Answer from the drawing. Dimensions are ordinates in mm from the lowest x, y and z of the part. Coordinates: 2 decimals unless noted, no trailing zeros. Order: outer loops, then holes, each group sorted by start corner. A loop starts at its lowest first (then second) coordinate and runs counter-clockwise, first axis right, second up.
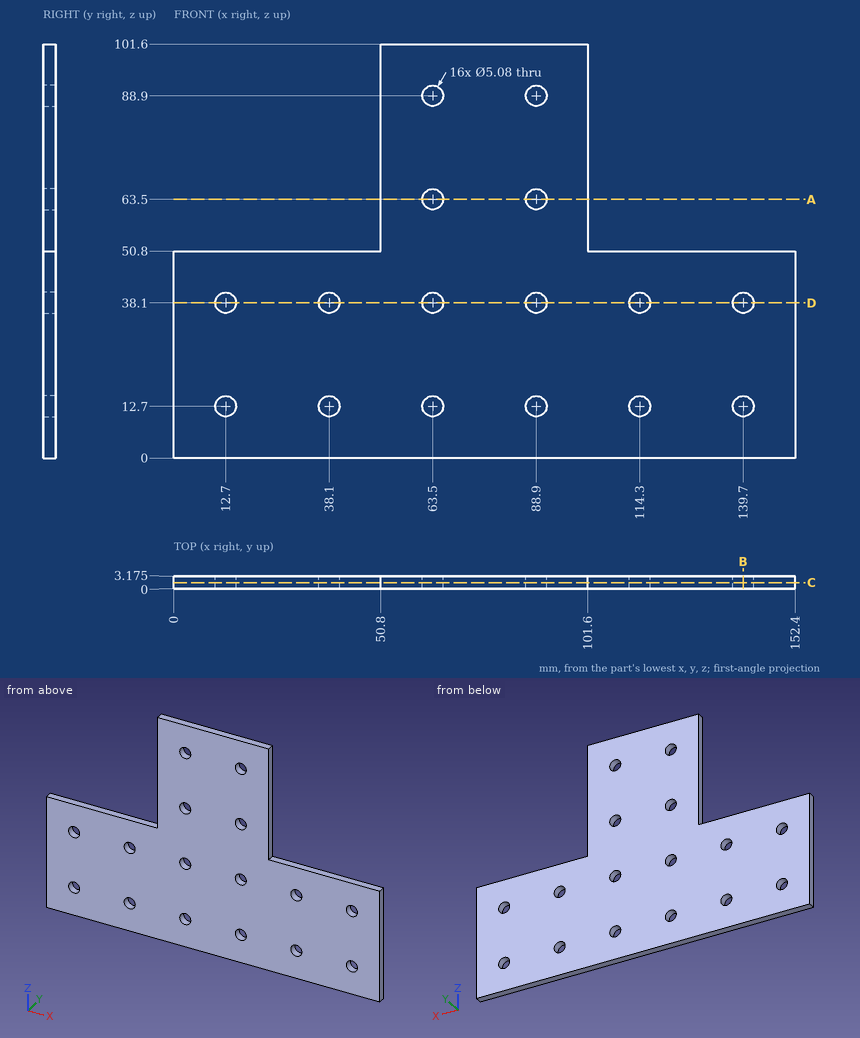
1. Flat-ended cylindrical pins translate along their axes: pin 1 (1 mm diameter, centred on x = 123.5, y = 1, fed in from +Z); pin 2 (3 mm diameter, centred on x = 139.7, z = 38.1, fed in from -Y); pin 3 (1.6 mm diameter, centred on y = 2, z = 68.5, fed in from +X). Find the tip coordinate at first contact, or state that the pin passes through.
2. Consider probe 1 along Z at (x, y) = (13, 1.25); probe 2 along Z at (x, y) = (89.5, 2.1); probe 3 along Z at (x, y) = (45, 1.9). Determine where each line is inside the solid, lowest interval first.
3. The part is cut by section B-B (x = 139.7). Determine the outline of the cut face in (y, z) (3 decimals), plus the area to 3 significant figures.
4. The part is cut by section D-D (z = 38.1). Determine the outline of the cut face in (x, y) (3 decimals).
5. The part is cut by section C-C (y = 1.55). Count the separate pieces of the cut face and the enclosed holes in it, plus the area to 4 significant figures.
6. The part is cut by section A-A (z = 63.5). Determine the outline of the cut face in (x, y) (3 decimals).
Worked out:
1. pin 1: stops at z = 50.8
1. pin 2: passes through
1. pin 3: stops at x = 101.6
2. probe 1: z = 0 to 10.18, 15.22 to 35.58, 40.62 to 50.8
2. probe 2: z = 0 to 10.23, 15.17 to 35.63, 40.57 to 61.03, 65.97 to 86.43, 91.37 to 101.6
2. probe 3: z = 0 to 50.8
3. outline: (0, 0) - (3.175, 0) - (3.175, 10.16) - (0, 10.16) - close; (0, 15.24) - (3.175, 15.24) - (3.175, 35.56) - (0, 35.56) - close; (0, 40.64) - (3.175, 40.64) - (3.175, 50.8) - (0, 50.8) - close
3. area: 129 mm2
4. outline: (0, 0) - (10.16, 0) - (10.16, 3.175) - (0, 3.175) - close; (15.24, 0) - (35.56, 0) - (35.56, 3.175) - (15.24, 3.175) - close; (40.64, 0) - (60.96, 0) - (60.96, 3.175) - (40.64, 3.175) - close; (66.04, 0) - (86.36, 0) - (86.36, 3.175) - (66.04, 3.175) - close; (91.44, 0) - (111.76, 0) - (111.76, 3.175) - (91.44, 3.175) - close; (116.84, 0) - (137.16, 0) - (137.16, 3.175) - (116.84, 3.175) - close; (142.24, 0) - (152.4, 0) - (152.4, 3.175) - (142.24, 3.175) - close
5. separate pieces: 1
5. enclosed holes: 16
5. area: 10,000 mm2
6. outline: (50.8, 0) - (60.96, 0) - (60.96, 3.175) - (50.8, 3.175) - close; (66.04, 0) - (86.36, 0) - (86.36, 3.175) - (66.04, 3.175) - close; (91.44, 0) - (101.6, 0) - (101.6, 3.175) - (91.44, 3.175) - close
